Autodesk Inventor part; units mm, degrees
ref_plane "YZ Plane" through (0, 0, 0) normal (1, 0, 0) x (0, 1, 0)
ref_plane "XZ Plane" through (0, 0, 0) normal (0, 1, 0) x (-1, 0, 0)
ref_plane "XY Plane" through (0, 0, 0) normal (0, 0, 1) x (1, 0, 0)
sketch "Sketch1" plane through (0, 0, 0) normal (0, 0, 1) x (1, 0, 0)
  line L0 (-12.7, -25.4) -> (12.7, -25.4)
  line L1 (12.7, -25.4) -> (12.7, 25.4)
  line L2 (12.7, 25.4) -> (-12.7, 25.4)
  line L3 (-12.7, 25.4) -> (-12.7, -25.4)
  line L4 (-12.7, -25.4) -> (12.7, 25.4) construction
  line L5 (12.7, -25.4) -> (-12.7, 25.4) construction
  line L6 (-10.16, -22.86) -> (10.16, -22.86)
  line L7 (10.16, -22.86) -> (10.16, 22.86)
  line L8 (10.16, 22.86) -> (-10.16, 22.86)
  line L9 (-10.16, 22.86) -> (-10.16, -22.86)
  line L10 (-10.16, -22.86) -> (10.16, 22.86) construction
  line L11 (10.16, -22.86) -> (-10.16, 22.86) construction
  point P0 (0, 0)
  dimension "d0" = 25.4
  dimension "d1" = 50.8
  dimension "d2" = 20.32
  dimension "d3" = 45.72
extrude "Extrusion1" add sketch "Sketch1" along normal mid plane 190.5
sketch "Sketch2" plane through (-12.7, 25.4, 95.25) normal (0, 1, 0) x (1, 0, 0)
  line L0 (0, 190.5) -> (0, 0)
  line L1 (25.4, 0) -> (0, 0)
  point P0 (12.7, 95.25)
  point P1 (12.7, 12.7)
  dimension "d6" = 12.7
  dimension "d7" = 12.7
hole "Hole1" at (0, 25.4, 82.55) direction (0, -1, 0) diameter 4.1402 end through all
pattern_linear "Rectangular Pattern1" count 7 spacing 25.4 along (0, 0, -1) of "Hole1"
sketch "Sketch3" plane through (12.7, -25.4, 95.25) normal (1, 0, 0) x (0, 0, -1)
  line L0 (0, 0) -> (0, 50.8)
  line L1 (190.5, 0) -> (0, 0)
  line L2 (190.5, 50.8) -> (190.5, 0)
  circle A0 centre (19.05, 19.05) radius 14.2748
  line L3 (190.5, 50.8) -> (0, 50.8)
  circle A1 centre (149.4019, 25.4) radius 2.0701
  circle A2 centre (177.8, 25.4) radius 2.0701
  point P0 (95.25, 25.4)
  dimension "d19" = 19.05
  dimension "d28" = 19.05
  dimension "d32" = 28.5496
  dimension "d35" = 25.4
  dimension "d36" = 12.7
  dimension "d37" = 28.3981
  dimension "d38" = 4.1402
  dimension "d39" = 4.1402
extrude "Extrusion2" cut sketch "Sketch3" against normal through all contours A0 | A1 | A2
properties part number "Diag_intake_hanger"
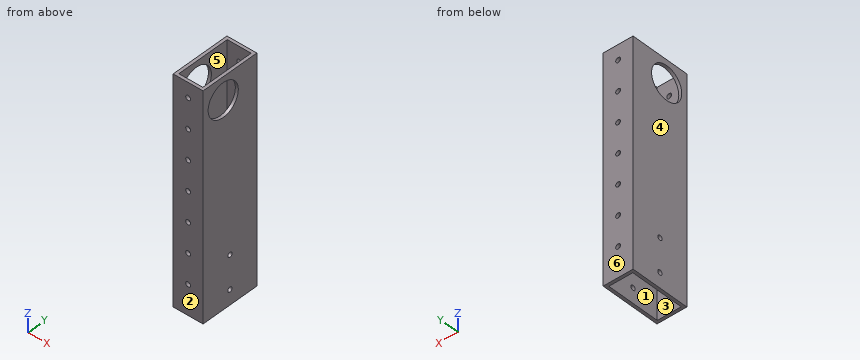
Geometry check sheet. Reference: the model listing, model coordinates, mm. Face numbers are marked on the shaded views. A direction names the side the tool comes from. Give positions to 0.01 mm unless a question says otherwise; leave off trailing zeros. Order: outer loops, then holes, each group sorted by start corner. A loop starts at its lowest first (then second) coordinate and runs counter-clockwise, first axis right, second up. Notation, with made-up numbers: M -34,-8.75 L -18,-8.75 A34 cw -18,29.25 Z; hole C 21,73 d7. An arc over 180 degrees is marked long. Use a Markdown table: item, result.
Item 1: Section check B-B (z = 6.35). Record the cut outline in (x, y), and give its area (3 significant figures).
Answers follow:
| item | result |
|---|---|
| outline | M -12.7,-25.4 L -2.07,-25.4 L -2.07,-22.86 L -10.16,-22.86 L -10.16,22.86 L -2.07,22.86 L -2.07,25.4 L -12.7,25.4 Z; M 2.07,-25.4 L 12.7,-25.4 L 12.7,25.4 L 2.07,25.4 L 2.07,22.86 L 10.16,22.86 L 10.16,-22.86 L 2.07,-22.86 Z |
| area | 340 mm2 |
Item 2: Depth check by flat-ended pin: P1, Ø5, axis at x = 0, z = 82.55, coming from the +Y side. Enter the tip coordinate at first touch or a pass-through.
Answers follow:
| item | result |
|---|---|
| P1 | stops at y = 25.4 |
Item 3: Draft check along X on the marked faces 3, 4, 5 and 6. Enter one of: +X half, -X half, draft (parallel to the pull), parting line (faces both ways), or undercut.
Answers follow:
| item | result |
|---|---|
| face 3 | undercut |
| face 4 | -X half |
| face 5 | undercut |
| face 6 | draft |
Item 4: Section check D-D (z = -40). Record the cut outline in (x, y).
Answers follow:
| item | result |
|---|---|
| outline | M -12.7,-25.4 L 12.7,-25.4 L 12.7,25.4 L -12.7,25.4 Z; hole M -10.16,-22.86 L 10.16,-22.86 L 10.16,22.86 L -10.16,22.86 Z |
Item 5: Section check C-C (y = -6.35). Record the cut outline in (x, z), and give its area (3 significant figures).
Answers follow:
| item | result |
|---|---|
| outline | M -12.7,-95.25 L -10.16,-95.25 L -10.16,61.93 L -12.7,61.93 Z; M -12.7,90.47 L -10.16,90.47 L -10.16,95.25 L -12.7,95.25 Z; M 10.16,-95.25 L 12.7,-95.25 L 12.7,61.93 L 10.16,61.93 Z; M 10.16,90.47 L 12.7,90.47 L 12.7,95.25 L 10.16,95.25 Z |
| area | 823 mm2 |
Item 6: Section check A-A (x = -5.25). Record the cut outline in (y, z), and give its area (3 significant figures).
Answers follow:
| item | result |
|---|---|
| outline | M -25.4,-95.25 L -22.86,-95.25 L -22.86,95.25 L -25.4,95.25 Z; M 22.86,-95.25 L 25.4,-95.25 L 25.4,95.25 L 22.86,95.25 Z |
| area | 968 mm2 |
Item 7: Tool access check on the marked faces 1 and 2. Record the directions out of +Z, -Z, +X, -X, +Y, -Y that give a thin tool (end or side, any length) a straight path to the whole face; none if there is none.
Answers follow:
| item | result |
|---|---|
| face 1 | +Z, -Z |
| face 2 | +Z, -Z, +X, -X, -Y |
Item 8: Material ranges on line 1 along Y through (x, z) = (-4, -1.5); line 2 along X through (y, z) = (6.5, -6.5); line 3 along X through (y, z) = (-24, 6), recorded low to high.
Answers follow:
| item | result |
|---|---|
| line 1 | y = -25.4 to -22.86, 22.86 to 25.4 |
| line 2 | x = -12.7 to -10.16, 10.16 to 12.7 |
| line 3 | x = -12.7 to -2.04, 2.04 to 12.7 |
